```python
from build123d import *

# Parameters (mm, degrees)
EXTRUDE_THIN_START                    = 2
EXTRUDE_THIN_HOLDER_WALLS_OUTLINE_W   = 69
EXTRUDE_THIN_HOLDER_WALLS_OUTLINE_H   = 39.4
EXTRUDE_THIN_HOLDER_WALLS_OUTLINE_W_2 = 67
EXTRUDE_THIN_HOLDER_WALLS_OUTLINE_H_2 = 37.4
EXTRUDE_THIN_HOLDER_WALLS_DEPTH       = 19.8
BOSS_EXTRUDE_START                    = 20.8
BATTERY_HOLDER_AREA_8_W               = 28.6
BATTERY_HOLDER_AREA_8_H               = 37.4
BATTERY_HOLDER_AREA_8_W_2             = 5
BATTERY_HOLDER_AREA_8_H_2             = 10
BOSS_EXTRUDE_HOLDER_TOP_DEPTH         = 1
CUT_EXTRUDE_START                     = 14.8
BATTERY_HOLDER_AREA_6_W               = 1
BATTERY_HOLDER_AREA_6_H               = 10
BATTERY_HOLDER_AREA_6_W_2             = 5
CUT_EXTRUDE_BATTERY_CABLE_DEPTH       = 7
BOSS_EXTRUDE_START_2                  = 2
BOSS_EXTRUDE_SLIDE_CLAMP_DEPTH        = 1.5
FILLET_SLIDE_CLAMP_SIZE               = 0.75
FILLET_HOLDER_EDGES_R                 = 2
BATTERY_HOLDER_AREA_6_2_W             = 1
BATTERY_HOLDER_AREA_6_2_H             = 7
EXTRUDE_THIN_HOLDER_CLIPS_DEPTH       = 12.8
BOSS_EXTRUDE_START_3                  = 14.8
BATTERY_HOLDER_AREA_6_3_W             = 3
BATTERY_HOLDER_AREA_6_3_H             = 7
BATTERY_HOLDER_AREA_6_3_W_2           = 1.2
BOSS_EXTRUDE_HOLDER_CLIP_BASES_DEPTH  = 3
CHAMFER_HOLDER_CLIP_BASES_SIZE        = 1.5
BATTERY_HOLDER_AREA_6_4_W             = 2.3
BATTERY_HOLDER_AREA_6_4_H             = 7
EXTRUDE_THIN_HOLDER_CLIP_HOOK_DEPTH   = 1.6
CHAMFER_HOLDER_CLIP_HOOK_SIZE         = 1.349017034
CHAMFER_HOLDER_CLIP_HOOK_SIZE2        = 2


with BuildPart() as part:
    # Extrude-Thin holder walls: read off the stored shape, not the designer's step
    # Extrude-Thin holder walls outline → Extrude-Thin holder walls (new body)
    with BuildSketch(Plane(origin=(0, 0, 0), x_dir=(1, 0, 0), z_dir=(0, 1, 0)).offset(EXTRUDE_THIN_START)):
        with Locations((0, -11.3)):
            Rectangle(EXTRUDE_THIN_HOLDER_WALLS_OUTLINE_W, EXTRUDE_THIN_HOLDER_WALLS_OUTLINE_H)
        with Locations((0, -11.3)):
            Rectangle(EXTRUDE_THIN_HOLDER_WALLS_OUTLINE_W_2, EXTRUDE_THIN_HOLDER_WALLS_OUTLINE_H_2, mode=Mode.SUBTRACT)
    extrude(amount=EXTRUDE_THIN_HOLDER_WALLS_DEPTH)

    # Battery holder area_8 → Boss-Extrude holder top (add)
    with BuildSketch(Plane(origin=(0, 0, 0), x_dir=(1, 0, 0), z_dir=(0, 1, 0)).offset(BOSS_EXTRUDE_START)):
        Polygon((0, -30), (0, 7.4), (-33.5, 7.4), (-33.5, 6.1), (-33.5, -6.3), (-28.5, -6.3), (-28.5, -16.3), (-33.5, -16.3), (-33.5, -28.7), (-33.5, -30), align=None)
        with Locations((14.3, -11.3)):
            Rectangle(BATTERY_HOLDER_AREA_8_W, BATTERY_HOLDER_AREA_8_H)
        Polygon((33.5, 7.4), (28.6, 7.4), (28.6, -30), (33.5, -30), (33.5, -14.8), (33.5, -7.8), align=None)
        with Locations((-31, -11.3)):
            Rectangle(BATTERY_HOLDER_AREA_8_W_2, BATTERY_HOLDER_AREA_8_H_2)
    extrude(amount=BOSS_EXTRUDE_HOLDER_TOP_DEPTH)

    # Battery holder area_6 → Cut-Extrude battery cable (cut)
    with BuildSketch(Plane(origin=(0, 0, 0), x_dir=(1, 0, 0), z_dir=(0, 1, 0)).offset(CUT_EXTRUDE_START)):
        with Locations((-34, -11.3)):
            Rectangle(BATTERY_HOLDER_AREA_6_W, BATTERY_HOLDER_AREA_6_H)
        with Locations((-31, -11.3)):
            Rectangle(BATTERY_HOLDER_AREA_6_W_2, BATTERY_HOLDER_AREA_6_H)
    extrude(amount=CUT_EXTRUDE_BATTERY_CABLE_DEPTH, mode=Mode.SUBTRACT)

    # Battery holder area_8 2 → Boss-Extrude slide clamp (add)
    with BuildSketch(Plane(origin=(0, 0, 0), x_dir=(1, 0, 0), z_dir=(0, 1, 0)).offset(BOSS_EXTRUDE_START_2)):
        Polygon((-36.5, -28.7), (-33.5, -28.7), (-33.5, -16.3), (-34.5, -16.3), (-34.5, -6.3), (-33.5, -6.3), (-33.5, 6.1), (-36.5, 6.1), align=None)
    extrude(amount=BOSS_EXTRUDE_SLIDE_CLAMP_DEPTH)

    # Fillet slide clamp
    # a fillet whose section is not a circle: 0.75 mm, written as the material it takes off along each edge
    with BuildSketch(Plane(origin=(-36.5, 2, -7.975), x_dir=(0, 1, 0), z_dir=(0, 0, 1))) as fillet_slide_clamp_piece_1:
        with BuildLine():
            add(Edge.make_bspline([(FILLET_SLIDE_CLAMP_SIZE, 0), (FILLET_SLIDE_CLAMP_SIZE * 0.831801948466, 0), (FILLET_SLIDE_CLAMP_SIZE * 0.663603896932, 0), (FILLET_SLIDE_CLAMP_SIZE * 0.292893218813, -FILLET_SLIDE_CLAMP_SIZE * 0.0716919198361), (FILLET_SLIDE_CLAMP_SIZE * 0.0716919198361, -FILLET_SLIDE_CLAMP_SIZE * 0.292893218813), (0, -FILLET_SLIDE_CLAMP_SIZE * 0.663603896932), (0, -FILLET_SLIDE_CLAMP_SIZE * 0.831801948466), (0, -FILLET_SLIDE_CLAMP_SIZE)], knots=[0, 0, 0, 0, 0, 0, 0.5, 0.5, 1, 1, 1, 1, 1, 1], degree=5))
            Line((0, -FILLET_SLIDE_CLAMP_SIZE), (0, 0))
            Line((0, 0), (FILLET_SLIDE_CLAMP_SIZE, 0))
        make_face()
    extrude(amount=38.55, mode=Mode.SUBTRACT)

    # Fillet holder edges
    fillet_holder_edges_edges = [part.edges().sort_by_distance(p)[0] for p in [
        (34.5, 21.8, 11.3),
        (0, 21.8, 31),
        (-34.5, 21.8, 23.65),
        (0, 21.8, -8.4),
        (-34.5, 21.8, -1.05),
    ]]
    fillet(fillet_holder_edges_edges, radius=FILLET_HOLDER_EDGES_R)



with BuildPart() as body_2:
    # Battery holder area_6 2 → Extrude-Thin holder clips (new body)
    with BuildSketch(Plane(origin=(0, 0, 0), x_dir=(1, 0, 0), z_dir=(0, 1, 0)).offset(EXTRUDE_THIN_START)):
        with Locations((38.2, -11.3)):
            Rectangle(BATTERY_HOLDER_AREA_6_2_W, BATTERY_HOLDER_AREA_6_2_H)
    extrude(amount=EXTRUDE_THIN_HOLDER_CLIPS_DEPTH)


with BuildPart() as part_1:
    add(part.part)

    add(body_2.part)  # Boss-Extrude holder clip bases merges body 2
    # Battery holder area_6 3 → Boss-Extrude holder clip bases (add)
    with BuildSketch(Plane(origin=(0, 0, 0), x_dir=(1, 0, 0), z_dir=(0, 1, 0)).offset(BOSS_EXTRUDE_START_3)):
        with Locations((36.2, -11.3)):
            Rectangle(BATTERY_HOLDER_AREA_6_3_W, BATTERY_HOLDER_AREA_6_3_H)
        with Locations((34.1, -11.3)):
            Rectangle(BATTERY_HOLDER_AREA_6_3_W_2, BATTERY_HOLDER_AREA_6_3_H)
    extrude(amount=-BOSS_EXTRUDE_HOLDER_CLIP_BASES_DEPTH)

    # Chamfer holder clip bases
    chamfer_holder_clip_bases_edges = [part_1.edges().sort_by_distance(p)[0] for p in [
        (37.7, 11.8, 11.3),
        (38.7, 14.8, 11.3),
    ]]
    chamfer(chamfer_holder_clip_bases_edges, length=CHAMFER_HOLDER_CLIP_BASES_SIZE)

    # Battery holder area_6 4 → Extrude-Thin holder clip hook (add)
    with BuildSketch(Plane(origin=(0, 0, 0), x_dir=(1, 0, 0), z_dir=(0, 1, 0)).offset(EXTRUDE_THIN_START)):
        with Locations((37.55, -11.3)):
            Rectangle(BATTERY_HOLDER_AREA_6_4_W, BATTERY_HOLDER_AREA_6_4_H)
    extrude(amount=EXTRUDE_THIN_HOLDER_CLIP_HOOK_DEPTH)

    # Chamfer holder clip hook
    chamfer_holder_clip_hook_edges = [part_1.edges().sort_by_distance(p)[0] for p in [
        (36.4, 2, 11.3),
    ]]
    chamfer_holder_clip_hook_side = [part_1.faces().sort_by_distance(p)[0] for p in [
        (36.4, 2.8, 11.3),
    ]]
    chamfer(chamfer_holder_clip_hook_edges, length=CHAMFER_HOLDER_CLIP_HOOK_SIZE, length2=CHAMFER_HOLDER_CLIP_HOOK_SIZE2, reference=chamfer_holder_clip_hook_side[0])


solid = part_1.part
```
Check sheet for the modelled part. Datum: model origin and axes. Units: mm. A direction names the side the tool comes from. Round coordinates to 2 decimals unless told otherwise and drop trailing zeros. Loops run counter-clockwise (first coordinate to the right, second up) from the corner with the lowest first, then second, coordinate; pieces in that order, holes last. Notation, with made-up numbers: (30.25, 31) -> (59.25, 31) arc R14 cw to (59.25, 36) -> close; hole circle Ø1 at (-40, 89). An arc over 180 degrees is marked (long way). Write item = value, one per line. Start each with the question number.
1) Sectioned sample at A-A, the plane y = 11. Record the cut outline in (x, z).
2) Sectioned sample at C-C, the plane y = 16.5. Record the cut outline in (x, z).
3) Release check for a two-part mould opening along Z. For faces 4 (the flat face through (0, 11, 30)), 5 (the cylindrical face through (0, 21, -8)), 6 (the flat face through (33.5, 11, 12)), 7 (the cylindrical face through (-33.93, 21.2, -1.15)) record: released by +Z, released by -Z, zero draft, split by the parting line, or undercut.
4) Gauge pin test, flat ends, axial feed: pin 1 Ø0.5 at (y, z) = (21.5, 12) entering from -X; pin 2 Ø0.5 at (x, z) = (-34, 12.5) entering from +Y; pin 3 Ø0.5 at (x, y) = (-36, 3) entering from -Z. Record the tip position at first contact, or that the pin passes through.
5) Thickness scan on probe 1 along X at (y, z) = (9, -6); probe 2 along Z at (x, y) = (-28, 17.25); probe 3 along Y at (x, z) = (11, 0). Record the ranges inside material, lowest first.
6) Set-up check for faces 1 (the flat face through (37.41, 2.67, 11.35)), 2 (the flat face through (0, 20.8, 11)), 3 (the flat face through (38, 10, 14.8)): record each of +Z, -Z, +X, -X, +Y, -Y from which the full face is reachable in a straight line by a thin tool's end or side.
7) Sectioned sample at B-B, the plane x = 19. Record the cut outline in (y, z), plus the area to 3 significant figures.
Results are:
q1.outline = (-34.5, -8.4) -> (34.5, -8.4) -> (34.5, 31) -> (-34.5, 31) -> close; (37, 7.8) -> (38.7, 7.8) -> (38.7, 14.8) -> (37, 14.8) -> close; hole (-33.5, -7.4) -> (33.5, -7.4) -> (33.5, 30) -> (-33.5, 30) -> close
q2.outline = (-34.5, -8.4) -> (34.5, -8.4) -> (34.5, 31) -> (-34.5, 31) -> (-34.5, 16.3) -> (-33.5, 16.3) -> (-33.5, 30) -> (33.5, 30) -> (33.5, -7.4) -> (-33.5, -7.4) -> (-33.5, 6.3) -> (-34.5, 6.3) -> close
q3.face_4 = undercut
q3.face_5 = released by -Z
q3.face_6 = undercut
q3.face_7 = zero draft
q4.pin_1 = -28.5
q4.pin_2 = 14.8
q4.pin_3 = -6.1
q5.probe_1 = -34.5 to -33.5, 33.5 to 34.5
q5.probe_2 = -8.4 to -7.4, 30 to 31
q5.probe_3 = 20.8 to 21.8
q6.face_1 = +Z, -Z, -Y
q6.face_2 = -Y
q6.face_3 = +Z, +X, +Y, -Y
q7.outline = (2, -8.4) -> (19.8, -8.4) arc R2 ccw to (21.8, -6.4) -> (21.8, 29) arc R2 ccw to (19.8, 31) -> (2, 31) -> (2, 30) -> (20.8, 30) -> (20.8, -7.4) -> (2, -7.4) -> close
q7.area = 75.3 mm^2
